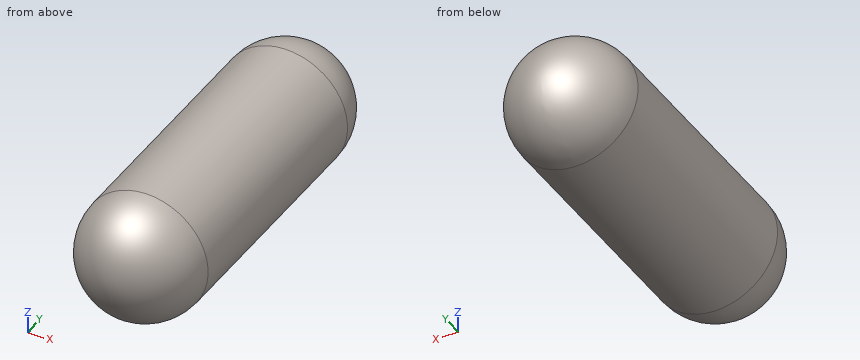
```python
from build123d import *

# Parameters (mm, degrees)
SKETCH1_R           = 50.8
BOSS_EXTRUDE1_DEPTH = 101.6


with BuildPart() as part:
    # Sketch1 → Boss-Extrude1 (new, symmetric)
    with BuildSketch(Plane(origin=(0, 0, 0), x_dir=(1, 0, 0), z_dir=(0, 1, 0))):
        with Locations(Location((0, 0, 0), (0, 0, 270))):
            Circle(SKETCH1_R)
    extrude(amount=BOSS_EXTRUDE1_DEPTH, both=True)

    # Sketch3 → Revolve1 (revolve)
    with BuildSketch(Plane(origin=(0, 0, 0), x_dir=(0, 0, -1), z_dir=(1, 0, 0)), mode=Mode.PRIVATE) as revolve1_sk:
        with BuildLine():
            Line((0, 101.6), (-50.8, 101.6))
            ThreePointArc((-50.8, 101.6), (-35.921024484, 137.521024484), (0, 152.4))
            Line((0, 152.4), (0, 101.6))
        make_face()
    revolve1 = revolve(revolve1_sk.sketch.rotate(Axis((0, 152.4, 0), (0, -1, 0)), 180), axis=Axis((0, 152.4, 0), (0, -1, 0)))

    # Mirror1: Revolve1 across plane
    add(revolve1.mirror(Plane.ZX))


solid = part.part
```
The model under review builds one solid part; all positions refer to its coordinate system, in mm. Give positions to 0.01 mm unless a question says otherwise; leave off trailing zeros. Write each loop counter-clockwise with the first axis right and the second up, starting at its lowest first coordinate (ties: lowest second). Pieces come first, ordered by that corner, then holes. Notation, with made-up numbers: (-24, 7) -> (-10, 7) arc R29 ccw to (-10, 34) -> close; hole circle Ø11 at (46.25, 24.25). An arc over 180 degrees is marked (long way). Put each result on its own line as item: value.
(1) We need section B-B, the plane x = 0. Give the boundary of the cut face in (y, z).
Results are:
outline: (-101.6, -50.8) -> (101.6, -50.8) arc R50.8 ccw to (101.6, 50.8) -> (-101.6, 50.8) arc R50.8 ccw to start
(2) For pin 1 Ø10 at (y, z) = (-87.5, 8.5) entering from +X; pin 2 Ø6 at (x, y) = (20.5, 77.5) entering from +Z; pin 3 Ø1.5 at (x, y) = (-16, 65) entering from +Z, all flat-tipped, find the tip position at first contact; note any pin that passes through.
Results are:
pin 1: x = 50.68
pin 2: z = 47.69
pin 3: z = 48.46
(3) We need section A-A, the plane y = -62.5. Give the boundary of the cut face in (x, z).
Results are:
outline: circle Ø101.6 at (0, 0)
(4) We need section C-C, the plane z = 0. Give the boundary of the cut face in (x, y).
Results are:
outline: (-50.8, -101.6) arc R50.8 ccw to (50.8, -101.6) -> (50.8, 101.6) arc R50.8 ccw to (-50.8, 101.6) -> close
(5) To check wall thickness, follow probe 1 along Z at (x, y) = (-15, 59); probe 2 along Z at (x, y) = (-42, 57); probe 3 along X at (y, z) = (-71, 43). State the ranges of each line that lie inside material, in increasing order. Write a range as from..to.
Results are:
probe 1: -48.53..48.53
probe 2: -28.58..28.58
probe 3: -27.05..27.05
